The model under review builds one solid part; all positions refer to its coordinate system, in mm. Face numbers are marked on the shaded views. A direction names the side the tool comes from. Coordinates: 2 decimals unless noted, no trailing zeros. Order: outer loops, then holes, each group sorted by start corner. A loop starts at its lowest first (then second) coordinate and runs counter-clockwise, first axis right, second up. Notation, with made-up numbers: M 89.5,47.5 L 144.5,47.5 A20 cw 144.5,78.5 Z; hole C 36,29 d5. An arc over 180 degrees is marked long. One line per item, written item: value.
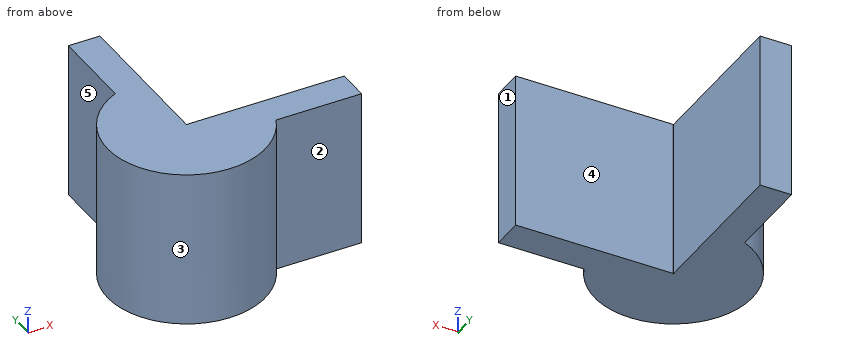
```python
from build123d import *

# Parameters (mm, degrees)
F1_DEPTH = 10


with BuildPart() as f1:
    # F0 (on Top) → F1 (new body)
    with BuildSketch(Plane.XY):
        with BuildLine():
            Line((-2, 10), (-2, 4.582576))
            ThreePointArc((-2, 4.582576), (-1.021548, 4.894532), (0, 5))
            Line((0, 5), (0, 10))
            Line((0, 10), (-2, 10))
        make_face()
        with BuildLine():
            Line((4.582576, -2), (10, -2))
            Line((10, -2), (10, 0))
            Line((10, 0), (5, 0))
            ThreePointArc((5, 0), (4.894532, -1.021548), (4.582576, -2))
        make_face()
        with BuildLine():
            Line((0, -2), (4.582576, -2))
            ThreePointArc((4.582576, -2), (4.894532, -1.021548), (5, 0))
            Line((5, 0), (0.024659, 0))
            ThreePointArc((0.024659, 0), (0.017436, -0.017436), (0, -0.024659))
            Line((0, -0.024659), (0, -2))
        make_face()
        with BuildLine():
            ThreePointArc((0, 5), (-1.021548, 4.894532), (-2, 4.582576))
            Line((-2, 4.582576), (-2, 0))
            Line((-2, 0), (-0.024659, 0))
            ThreePointArc((-0.024659, 0), (-0.017436, 0.017436), (0, 0.024659))
            Line((0, 0.024659), (0, 5))
        make_face()
        with BuildLine():
            ThreePointArc((-2, 4.582576), (-3.535534, -3.535534), (4.582576, -2))
            Line((4.582576, -2), (0, -2))
            Line((0, -2), (0, -0.024659))
            ThreePointArc((0, -0.024659), (-0.017436, -0.017436), (-0.024659, 0))
            Line((-0.024659, 0), (-2, 0))
            Line((-2, 0), (-2, 4.582576))
        make_face()
    extrude(amount=F1_DEPTH)


solid = f1.part
```
(1) Insertion check: pin 1 Ø3 at (y, z) = (6, 5) entering from -X; pin 2 Ø2.5 at (y, z) = (7.5, 6.5) entering from -X; pin 3 Ø1 at (y, z) = (3, 3) entering from +X. Each pin has a flat end and moves straight along its axis. Give the tip position at first contact, or say it passes through.
Geometry results:
pin 1: stops at x = -2.18
pin 2: stops at x = -2
pin 3: stops at x = 0
(2) We need section B-B, the plane x = 8.25. State the section outline as (y, z) points, plus the area to 3 significant figures.
Geometry results:
outline: M -2,0 L 0,0 L 0,10 L -2,10 Z
area: 20.0 mm2
(3) We need section C-C, the plane y = -2.75. State the section outline as (x, z) points.
Geometry results:
outline: M -4.18,0 L 4.18,0 L 4.18,10 L -4.18,10 Z
(4) For L1, parallel to X at y = 6.5, z = 2; L2, parallel to Y at x = 3.5, z = 3.5, list the stretches that pass through material, from the lowest coordinate up.
Geometry results:
L1: x = -2 to 0
L2: y = -3.57 to 0
(5) Tool access review of the marked faces 1, 2, 3, 4 and 5: name each direction out of +Z, -Z, +X, -X, +Y, -Y from which nothing blocks a thin tool from reaching the whole face with its end or side.
Geometry results:
face 1: +Z, -Z, +X, +Y, -Y
face 2: +Z, -Z, +X, -Y
face 3: +Z, -Z
face 4: +Z, -Z, +X, +Y
face 5: +Z, -Z, -X, +Y
